Read the model definition and answer for the solid it produces. Units are mm, in the model's axes. Face numbers are marked on the shaded views. A direction names the side the tool comes from. Give positions to 0.01 mm unless a question says otherwise; leave off trailing zeros. Write each loop counter-clockwise with the first axis right and the second up, starting at its lowest first coordinate (ties: lowest second). Pieces come first, ordered by that corner, then holes. Notation, with made-up numbers: (17.25, 10.25) - (38.25, 10.25) arc R19 ccw to (38.25, 46.25) - close; hole circle Ø6 at (-5.75, -28.75). An arc over 180 degrees is marked (long way). Answer as CSV lines item,"result".
```python
from build123d import *

# Parameters (mm, degrees)
SKETCH1_W               = 50
SKETCH1_H               = 20
BOSS_EXTRUDE1_DEPTH     = 15
CUT_EXTRUDE1_DEPTH      = 54.150729064
CUT_EXTRUDE1_DEPTH_BACK = 54.150729064
CUT_EXTRUDE2_DEPTH      = 15
SKETCH4_R               = 2
CUT_EXTRUDE3_DEPTH      = 10


with BuildPart() as part:
    # Sketch1 → Boss-Extrude1 (new body)
    with BuildSketch(Plane.XY):
        Rectangle(SKETCH1_W, SKETCH1_H)
    extrude(amount=BOSS_EXTRUDE1_DEPTH)

    # Sketch2 → Cut-Extrude1 (cut, two sides: drawn at the far end of the back side and taken through both)
    with BuildSketch(Plane(origin=(25, 0, 0), x_dir=(0, 0, -1), z_dir=(1, 0, 0)).offset(-CUT_EXTRUDE1_DEPTH_BACK)):
        Polygon((59.925140333, -12.996257017), (0, -10), (-15, -9.25), (-74.925140333, -6.253742983), (-80.917654366, -126.104023649), (53.932626299, -132.846537682), align=None)
    extrude(amount=CUT_EXTRUDE1_DEPTH + CUT_EXTRUDE1_DEPTH_BACK, mode=Mode.SUBTRACT)

    # Sketch3 → Cut-Extrude2 (cut)
    with BuildSketch(Plane(origin=(0, 0, 0), x_dir=(-1, 0, 0), z_dir=(0, 0, -1))):
        with BuildLine():
            Line((-16, 10), (16, 10))
            ThreePointArc((16, 10), (0, -6), (-16, 10))
        make_face()
    extrude(amount=-CUT_EXTRUDE2_DEPTH, mode=Mode.SUBTRACT)

    # Sketch4 → Cut-Extrude3 (cut)
    with BuildSketch(Plane(origin=(0, 10, 0), x_dir=(1, 0, 0), z_dir=(0, 1, 0))):
        with Locations(Location((20.5, -7.5, 0), (0, 0, 270))):
            Circle(SKETCH4_R)
    cut_extrude3 = extrude(amount=-CUT_EXTRUDE3_DEPTH, mode=Mode.SUBTRACT)

    # Mirror1: Cut-Extrude3 across plane
    add(cut_extrude3.mirror(Plane(origin=(0, 0, 0), x_dir=(0, 0, 1), z_dir=(1, 0, 0))), mode=Mode.SUBTRACT)


solid = part.part
```
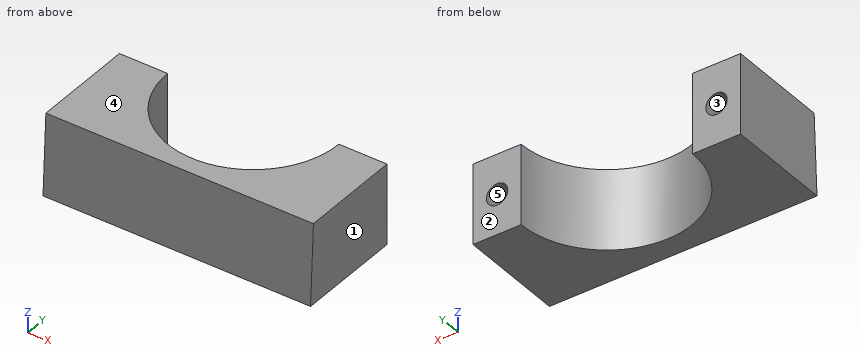
(1) A cutting plane is placed at C-C (z = 8.75). Write down the section's boundary in (x, y), and give its area (3 significant figures).
Worked out:
outline,"(-25, -9.56) - (25, -9.56) - (25, 10) - (22.06, 10) - (22.06, 0) - (18.94, 0) - (18.94, 10) - (16, 10) arc R16 cw to (-16, 10) - (-18.94, 10) - (-18.94, 0) - (-22.06, 0) - (-22.06, 10) - (-25, 10) - close"
area,"514 mm^2"
(2) A cutting plane is placed at B-B (x = 20.5). Write down the section's boundary in (y, z).
Worked out:
outline,"(-10, 0) - (10, 0) - (10, 5.5) - (0, 5.5) - (0, 9.5) - (10, 9.5) - (10, 15) - (-9.25, 15) - close"
(3) Each of these flat-tipped pins is pushed along its axis until it touches: P1, Ø5, axis at x = 19.5, z = 9.5, coming from the -Y side; P2, Ø3.5, axis at x = -20.5, z = 7.5, coming from the -Y side. Where does it stop, or does it pass through?
Worked out:
P1,"stops at y = -9.65"
P2,"stops at y = -9.71"
(4) The mould has two halves that part along X. Classify the marked faces 1, 2 and 3: +X half, -X half, draft (parallel to the pull), parting line (faces both ways), or undercut.
Worked out:
face 1,"+X half"
face 2,"draft"
face 3,"undercut"
(5) For the marked faces 4 and 5, determine the directions among +Z, -Z, +X, -X, +Y, -Y from which every point of the face is accessible in a straight line to the end or side of a thin tool.
Worked out:
face 4,"+Z, +X, -X, +Y, -Y"
face 5,"+Y"
(6) A cutting plane is placed at D-D (y = -2.5). Write down the section's boundary in (x, z), and give its area (3 significant figures).
Worked out:
outline,"(-25, 0) - (-9.99, 0) - (-9.99, 15) - (-25, 15) - close; (9.99, 0) - (25, 0) - (25, 15) - (9.99, 15) - close"
area,"450 mm^2"
(7) A cutting plane is placed at A-A (y = 5.75). Write down the section's boundary in (x, z).
Worked out:
outline,"(-25, 0) - (-15.43, 0) - (-15.43, 15) - (-25, 15) - close; (15.43, 0) - (25, 0) - (25, 15) - (15.43, 15) - close; hole circle Ø4 at (-20.5, 7.5); hole circle Ø4 at (20.5, 7.5)"
(8) Find the intervals of material crossed by L1, parallel to Z at x = -20.5, y = 5; L2, parallel to X at y = 3, z = 5.75; L3, parallel to X at y = 9, z = 9, in increasing order.
Worked out:
L1,"z = 0 to 5.5, 9.5 to 15"
L2,"x = -25 to -21.47, -19.53 to -14.39, 14.39 to 19.53, 21.47 to 25"
L3,"x = -25 to -21.82, -19.18 to -15.97, 15.97 to 19.18, 21.82 to 25"
